```python
from build123d import *

# Parameters (mm, degrees)
BOSS_EXTRUDE1_DEPTH     = 12.5
CUT_EXTRUDE1_DEPTH      = 122.726127023
CUT_EXTRUDE1_DEPTH_BACK = 122.726127023
SKETCH3_R               = 2.5
SKETCH2_W               = 17
SKETCH2_H               = 60
BOSS_EXTRUDE2_DEPTH     = 3
FILLET1_R               = 3


with BuildPart() as part:
    # Sketch1 → Boss-Extrude1 (new body)
    with BuildSketch(Plane(origin=(0, 0, 0), x_dir=(0, 0, -1), z_dir=(1, 0, 0))):
        Polygon((42, 78), (-42, 78), (-42, 0), (-45, 0), (-45, 81), (45, 81), (45, 0), (42, 0), align=None)
    extrude(amount=BOSS_EXTRUDE1_DEPTH)

    # Sketch3 → Cut-Extrude1 (cut, two sides: drawn at the far end of the back side and taken through both)
    with BuildSketch(Plane.XY.offset(45).offset(-CUT_EXTRUDE1_DEPTH_BACK)):
        with Locations((6.25, 71)):
            Circle(SKETCH3_R)
        with Locations((6.25, 7)):
            Circle(SKETCH3_R)
    extrude(amount=CUT_EXTRUDE1_DEPTH + CUT_EXTRUDE1_DEPTH_BACK, mode=Mode.SUBTRACT)

    # Sketch2 → Boss-Extrude2 (add)
    with BuildSketch(Plane(origin=(0, 81, 0), x_dir=(1, 0, 0), z_dir=(0, 1, 0))):
        with Locations((-8.5, 7.794002847)):
            Rectangle(SKETCH2_W, SKETCH2_H)
    extrude(amount=-BOSS_EXTRUDE2_DEPTH)

    # Fillet1
    fillet1_edges = [part.edges().sort_by_distance(p)[0] for p in [
        (0, 79.5, -37.794002847),
        (0, 79.5, 22.205997153),
    ]]
    fillet(fillet1_edges, radius=FILLET1_R)


solid = part.part
```
Model file for the job. Use its own axes, mm. A direction names the side the tool comes from. Coordinates: 2 decimals unless noted, no trailing zeros. Loops run counter-clockwise (first coordinate to the right, second up) from the corner with the lowest first, then second, coordinate; pieces in that order, holes last. Notation, with made-up numbers: (71, 17.5) -> (77, 17.5) arc R31 cw to (77, 54.5) -> close; hole circle Ø4 at (45, 48). An arc over 180 degrees is marked (long way). Answer as a JSON object with one key per item and string values.
Q1. Cut at B-B (x = 6.25). List the corners of the cut face in (y, z).
Report:
{"outline": "(0, -45) -> (4.5, -45) -> (4.5, -42) -> (0, -42) -> close; (0, 42) -> (4.5, 42) -> (4.5, 45) -> (0, 45) -> close; (9.5, -45) -> (68.5, -45) -> (68.5, -42) -> (9.5, -42) -> close; (9.5, 42) -> (68.5, 42) -> (68.5, 45) -> (9.5, 45) -> close; (73.5, -45) -> (81, -45) -> (81, 45) -> (73.5, 45) -> (73.5, 42) -> (78, 42) -> (78, -42) -> (73.5, -42) -> close"}
Q2. Cut at D-D (z = 30). List the corners of the cut face in (x, y), and give its area (3 significant figures).
Report:
{"outline": "(0, 78) -> (12.5, 78) -> (12.5, 81) -> (0, 81) -> close", "area": "37.5 mm2"}
Q3. 3-axis set-ups, long thin cutter, end or side, ignore diameter. For faces 1 (the flat face through (-2, 78, -1)), 2 (the flat face through (-10, 80, -37.794)), 3 (the flat face through (0, 47, 43)): which of +Z, -Z, +X, -X, +Y, -Y reach the whole face in a straight line?
Report:
{"face 1": "+X, -X, -Y", "face 2": "-Z, -X, +Y, -Y", "face 3": "+Z, -X, +Y, -Y"}
Q4. Probe probe 1 along Y at (x, z) = (6.25, 43.7); probe 2 along Z at (x, y) = (9.5, 68); probe 3 along X at (y, z) = (71, 43). List the from-to ranges inside material, lowest first.
Report:
{"probe 1": "y = 0 to 4.5, 9.5 to 68.5, 73.5 to 81", "probe 2": "z = -45 to -42, 42 to 45", "probe 3": "x = 0 to 3.75, 8.75 to 12.5"}
Q5. Cut at A-A (y = 71). List the corners of the cut face in (x, z).
Report:
{"outline": "(0, -45) -> (3.75, -45) -> (3.75, -42) -> (0, -42) -> close; (0, 42) -> (3.75, 42) -> (3.75, 45) -> (0, 45) -> close; (8.75, -45) -> (12.5, -45) -> (12.5, -42) -> (8.75, -42) -> close; (8.75, 42) -> (12.5, 42) -> (12.5, 45) -> (8.75, 45) -> close"}
Q6. Flat gauge pins, fed straight in: P1, Ø3.5, axis at y = 46.5, z = -42.5, coming from the -X side; P2, Ø8, axis at y = 20, z = -35.5, coming from the +X side; P3, Ø1.5, axis at x = -11, y = 79.5, coming from the +Z side; P4, Ø15, axis at x = -9.5, z = 20.5, coming from the -Y side. Where does each tip first touch, or does it go through?
Report:
{"P1": "stops at x = 0", "P2": "passes through", "P3": "stops at z = 22.21", "P4": "stops at y = 78"}
Q7. Cut at C-C (z = -8.5). List the corners of the cut face in (x, y).
Report:
{"outline": "(-17, 78) -> (12.5, 78) -> (12.5, 81) -> (-17, 81) -> close"}
Q8. Pull direction Z, two halves, no side cores. Call faces 4 (the flat face through (6, 0, -44)), 5 (the flat face through (6, 38, -42)), 6 (the flat face through (-10, 80, 22.206)): released by +Z, released by -Z, zero draft, split by the parting line, or undercut.
Report:
{"face 4": "zero draft", "face 5": "undercut", "face 6": "released by +Z"}
